from build123d import *

# Parameters (mm, degrees)
F0_R     = 23.495
F0_R_2   = 19.05
F1_DEPTH = 6.35
F2_DEPTH = 119.14632
F4_D     = 3.6576
F4_DEPTH = 12.7
F4_TIP   = 1.0988539001
F5_R     = 11.43
F6_DEPTH = 25.4
F7_R     = 11.90625
F8_DEPTH = 0.381


with BuildPart() as f1:
    # F0 (on Top) → F1 (new body)
    with BuildSketch(Plane.XY):
        Circle(F0_R)
        Circle(F0_R_2, mode=Mode.SUBTRACT)
    extrude(amount=F1_DEPTH)

    # F0 (on Top) → F2 (join)
    with BuildSketch(Plane.XY):
        Circle(F0_R_2)
    extrude(amount=F2_DEPTH)

    # F4
    with Locations(Plane.XY.offset(119.14632)):
        with Locations((0, 0)):
            Hole(F4_D / 2, depth=F4_DEPTH)
            with Locations((0, 0, -(F4_DEPTH + F4_TIP / 2))):  # 118° drill point
                Cone(0, F4_D / 2, F4_TIP, mode=Mode.SUBTRACT)

    # F5 (on Front) → F6 (cut, symmetric)
    with BuildSketch(Plane.XZ):
        with Locations((0, 50.8)):
            Circle(F5_R)
    extrude(amount=F6_DEPTH, both=True, mode=Mode.SUBTRACT)

    # F7 (on face) → F8 (cut)
    with BuildSketch(Plane(origin=(0, 0, 0), x_dir=(1, 0, 0), z_dir=(0, 0, -1))):
        Circle(F7_R)
    extrude(amount=-F8_DEPTH, mode=Mode.SUBTRACT)


solid = f1.part
The model under review builds one solid part; all positions refer to its coordinate system, in mm. A direction names the side the tool comes from. Coordinates: 2 decimals unless noted, no trailing zeros. Write each loop counter-clockwise with the first axis right and the second up, starting at its lowest first coordinate (ties: lowest second). Pieces come first, ordered by that corner, then holes. Notation, with made-up numbers: (61, 74) -> (97, 74) arc R17 ccw to (97, 82) -> close; hole circle Ø1 at (44.5, 27). An arc over 180 degrees is marked (long way). Answer in a Markdown table with one row per item.
1. We need section C-C, the plane x = -8. State the section outline as (y, z) points, and give its area (3 significant figures).
Answers below:
| item | result |
|---|---|
| outline | (-22.09, 0) -> (-8.82, 0) -> (-8.82, 0.38) -> (8.82, 0.38) -> (8.82, 0) -> (22.09, 0) -> (22.09, 6.35) -> (17.29, 6.35) -> (17.29, 42.64) -> (-17.29, 42.64) -> (-17.29, 6.35) -> (-22.09, 6.35) -> close; (-17.29, 58.96) -> (17.29, 58.96) -> (17.29, 119.15) -> (-17.29, 119.15) -> close |
| area | 3,610 mm^2 |
2. We need section D-D, the plane x = -13. State the section outline as (y, z) points.
Answers below:
| item | result |
|---|---|
| outline | (-19.57, 0) -> (19.57, 0) -> (19.57, 6.35) -> (13.92, 6.35) -> (13.92, 119.15) -> (-13.92, 119.15) -> (-13.92, 6.35) -> (-19.57, 6.35) -> close |
3. Draft analysis for pull direction X (two halves, no side actions). For faces 4 (the cylindrical face through (-5.093, -22.936, 3.131)), 5 (the cylindrical face through (1.451, -1.113, 112.707)), 6 (the flat face through (-0.1, 19.3, 6.35)), state which applies: +X half, -X half, draft (parallel to the pull), parting line (faces both ways), or undercut.
Answers below:
| item | result |
|---|---|
| face 4 | parting line |
| face 5 | undercut |
| face 6 | draft |
4. For faces 1 (the cylindrical face through (-11.42, -0.27, 51.3)), 2 (the cylindrical face through (-9.45, 7.24, 0.19)), 3 (the cylindrical face through (-19.03, 0.84, 61.96)), list the 3-axis set-ups (+Z, -Z, +X, -X, +Y, -Y) from which the entire face can be reached by the end or side of a thin tool; tool diameter is ignored.
Answers below:
| item | result |
|---|---|
| face 1 | +Y, -Y |
| face 2 | -Z |
| face 3 | +Z |
5. Wall thickness on probe 1 along Y at (x, z) = (0, 109); probe 2 along Z at (x, y) = (0.5, 4); probe 3 along Z at (x, y) = (0, 0): over which ranges is each line inside the solid? List them lowest first. Write a range as [from, to].
Answers below:
| item | result |
|---|---|
| probe 1 | y = [-19.05, -1.83], [1.83, 19.05] |
| probe 2 | z = [0.38, 39.38], [62.22, 119.15] |
| probe 3 | z = [0.38, 39.37], [62.23, 105.35] |
6. Clearance check with flat-ended pins moving along their axes: pin 1 Ø18.5 at (x, z) = (0, 50.8) entering from +Y; pin 2 Ø3 at (y, z) = (-6.5, 47.5) entering from -X; pin 3 Ø2 at (y, z) = (-1, 89) entering from -X; pin 4 Ø6 at (y, z) = (-9.5, 98.5) entering from +X. State where each tip first meets the part, or that it passes through.
Answers below:
| item | result |
|---|---|
| pin 1 | passes through |
| pin 2 | stops at x = -18.38 |
| pin 3 | stops at x = -19.05 |
| pin 4 | stops at x = 17.91 |
7. We need section A-A, the plane z = 50.8. State the section outline as (x, y) points.
Answers below:
| item | result |
|---|---|
| outline | (-11.43, -15.24) -> (-11.43, 15.24) arc R19.05 ccw to start; (11.43, -15.24) arc R19.05 ccw to (11.43, 15.24) -> close |
8. We need section B-B, the plane y = 7.5. State the section outline as (x, z) points.
Answers below:
| item | result |
|---|---|
| outline | (-22.27, 0) -> (-9.25, 0) -> (-9.25, 0.38) -> (9.25, 0.38) -> (9.25, 0) -> (22.27, 0) -> (22.27, 6.35) -> (17.51, 6.35) -> (17.51, 119.15) -> (-17.51, 119.15) -> (-17.51, 6.35) -> (-22.27, 6.35) -> close; hole circle Ø22.86 at (0, 50.8) |
